Study the drawing (mm; zero at the part's minimum x, y, z) and answer. Coordinates: 2 decimals unless noted, no trailing zeros. Order: outer loops, then holes, each group sorted by start corner. A loop starts at its lowest first (then second) coordinate and runs counter-clockwise, first axis right, second up.
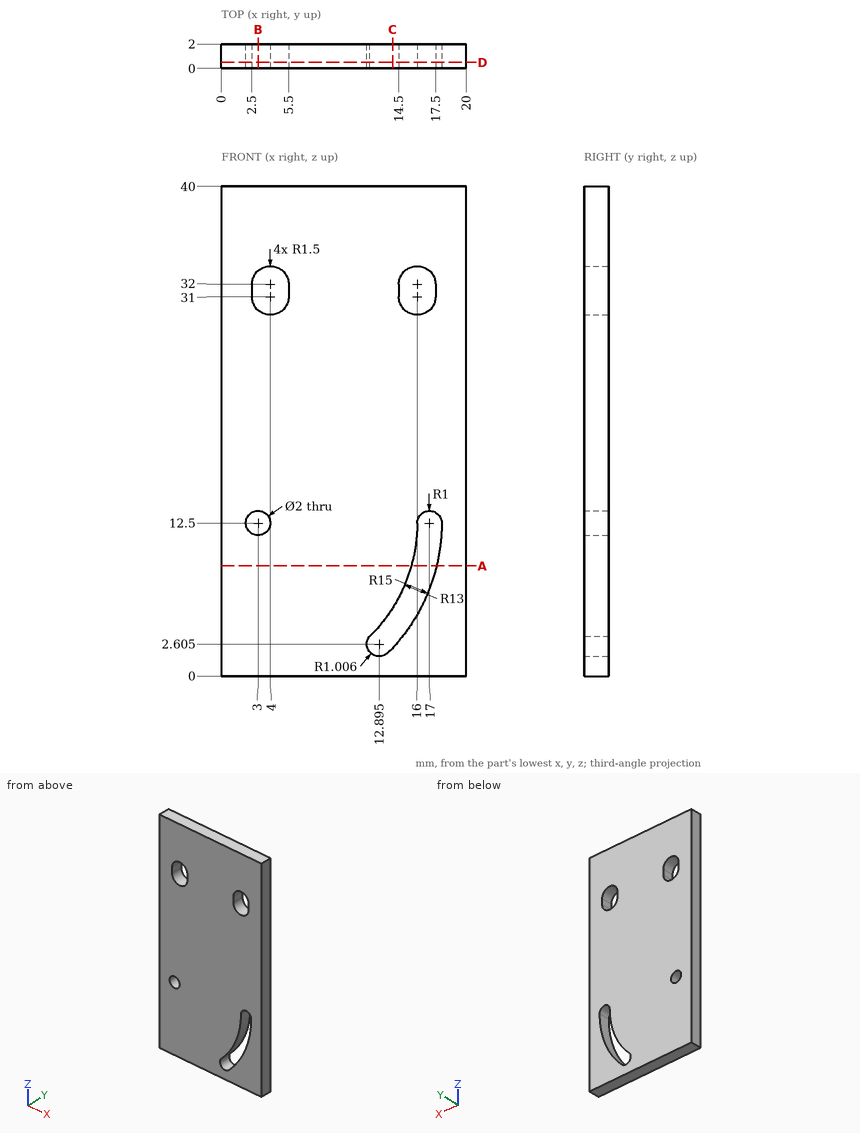
1) Straight lines are drawn through the part: line 1 (X direction, y = 0.95, z = 12.5); line 2 (Z direction, x = 3, y = 1.4); line 3 (X direction, y = 1, z = 30). For each, find the intervals that lie inside material, in ascending order.
A:
line 1: x = 0 to 2, 4 to 16, 18 to 20
line 2: z = 0 to 11.5, 13.5 to 29.88, 33.12 to 40
line 3: x = 0 to 2.88, 5.12 to 14.88, 17.12 to 20
2) A cutting plane is placed at C-C, the plane x = 14. Determine the outline of the cut face in (y, z).
A:
outline: (0, 0) - (2, 0) - (2, 2.3) - (0, 2.3) - close; (0, 5.57) - (2, 5.57) - (2, 40) - (0, 40) - close
3) A cutting plane is placed at A-A, the plane z = 9. Determine the outline of the cut face in (x, y).
A:
outline: (0, 0) - (15.52, 0) - (15.52, 2) - (0, 2) - close; (17.59, 0) - (20, 0) - (20, 2) - (17.59, 2) - close
4) A cutting plane is placed at B-B, the plane x = 3. Determine the outline of the cut face in (y, z).
A:
outline: (0, 0) - (2, 0) - (2, 11.5) - (0, 11.5) - close; (0, 13.5) - (2, 13.5) - (2, 29.88) - (0, 29.88) - close; (0, 33.12) - (2, 33.12) - (2, 40) - (0, 40) - close
5) A cutting plane is placed at D-D, the plane y = 0.5. Determine the outline of the cut face in (x, z) (1 decimal).
A:
outline: (0, 0) - (20, 0) - (20, 40) - (0, 40) - close; hole circle Ø2 at (3, 12.5); hole (2.5, 31) arc R1.5 ccw to (5.5, 31) - (5.5, 32) arc R1.5 ccw to (2.5, 32) - close; hole (12.1, 3.2) arc R1 ccw to (13.6, 1.9) arc R15 ccw to (18, 12.5) arc R1 ccw to (16, 12.5) arc R13 cw to start; hole (14.5, 31) arc R1.5 ccw to (17.5, 31) - (17.5, 32) arc R1.5 ccw to (14.5, 32) - close
